Geometry: see drawing. Coordinates: mm, zero at the bounding-box minimum. Coordinates: 2 decimals unless noted, no trailing zeros. Write each loop counter-clockwise with the first axis right and the second up, starting at its lowest first coordinate (ties: lowest second). Pieces come first, ordered by that corner, then holes. Notation, with made-up numbers: (-30.5, 5) - (20.5, 5) arc R17 ccw to (20.5, 36) - close; hole circle Ø10 at (65.5, 8.5). An arc over 180 degrees is marked (long way). One line per question, with ' | ' between items. Start each with the question number.
Q1. Cut plane A-A, the plane x = 41.5. Return loops of the section in (y, z).
Q2. Cut plane D-D, the plane x = 7.5. Return loops of the section in (y, z) (1 decimal).
Q3. Cut plane B-B, the plane y = 1.8. Return loops of the section in (x, z) (1 decimal).
Q4. Line query: line 1 (X direction, y = 0.45, z = 25) (1 decimal); line 2 (Z direction, x = 16.5, y = 1.45) (1 decimal); line 3 (Z direction, x = 36.5, y = 2.1) (1 decimal). Output: solid intervals per line, ascending.
Q5. Cut plane C-C, the plane z = 20.5. Return loops of the section in (x, y).
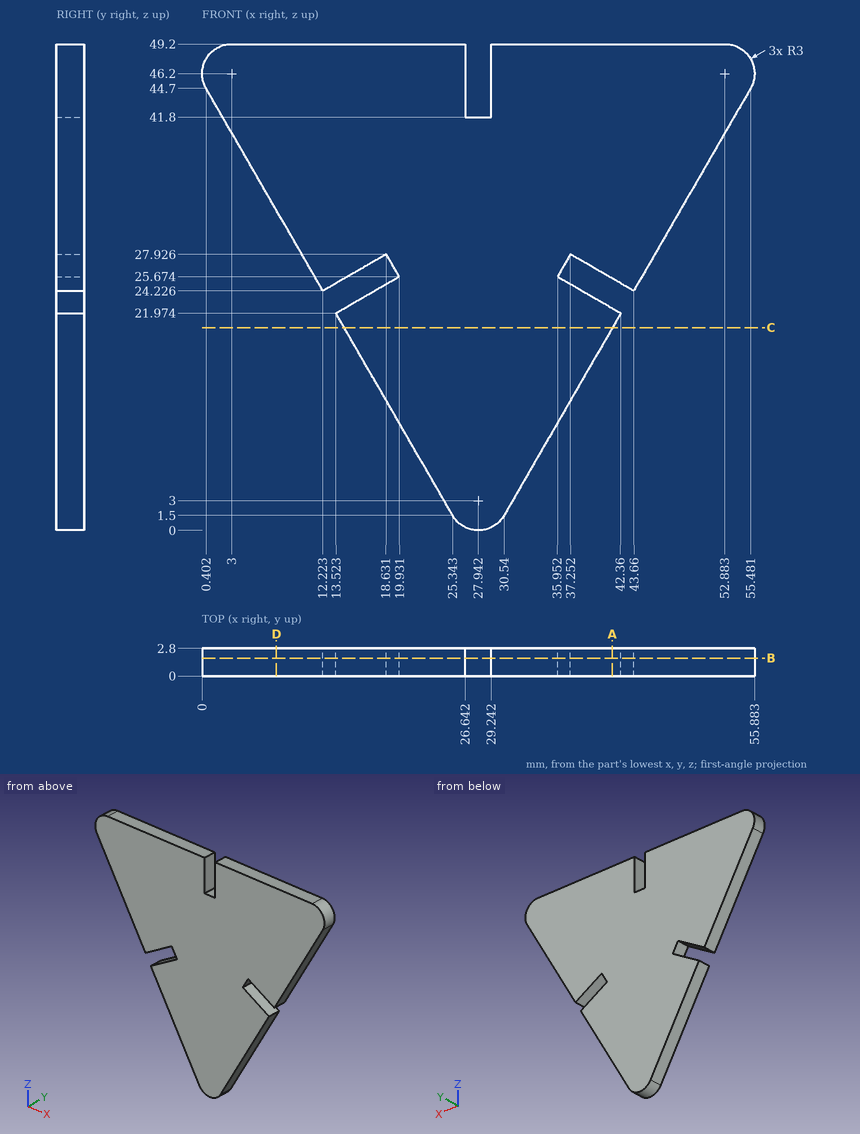
Reply:
1) outline: (0, 20.48) - (2.8, 20.48) - (2.8, 22.47) - (0, 22.47) - close; (0, 25.47) - (2.8, 25.47) - (2.8, 49.2) - (0, 49.2) - close
2) outline: (0, 32.4) - (2.8, 32.4) - (2.8, 49.2) - (0, 49.2) - close
3) outline: (0.4, 44.7) - (12.2, 24.2) - (18.6, 27.9) - (19.9, 25.7) - (13.5, 22) - (25.3, 1.5) arc R3 ccw to (30.5, 1.5) - (42.4, 22) - (36, 25.7) - (37.3, 27.9) - (43.7, 24.2) - (55.5, 44.7) arc R3 ccw to (52.9, 49.2) - (29.2, 49.2) - (29.2, 41.8) - (26.6, 41.8) - (26.6, 49.2) - (3, 49.2) arc R3 ccw to start
4) line 1: x = 11.8 to 13.6, 18.8 to 37.1, 42.3 to 44.1 | line 2: z = 16.8 to 23.7, 26.7 to 49.2 | line 3: z = 11.8 to 25.4, 26.6 to 49.2
5) outline: (14.37, 0) - (41.51, 0) - (41.51, 2.8) - (14.37, 2.8) - close
